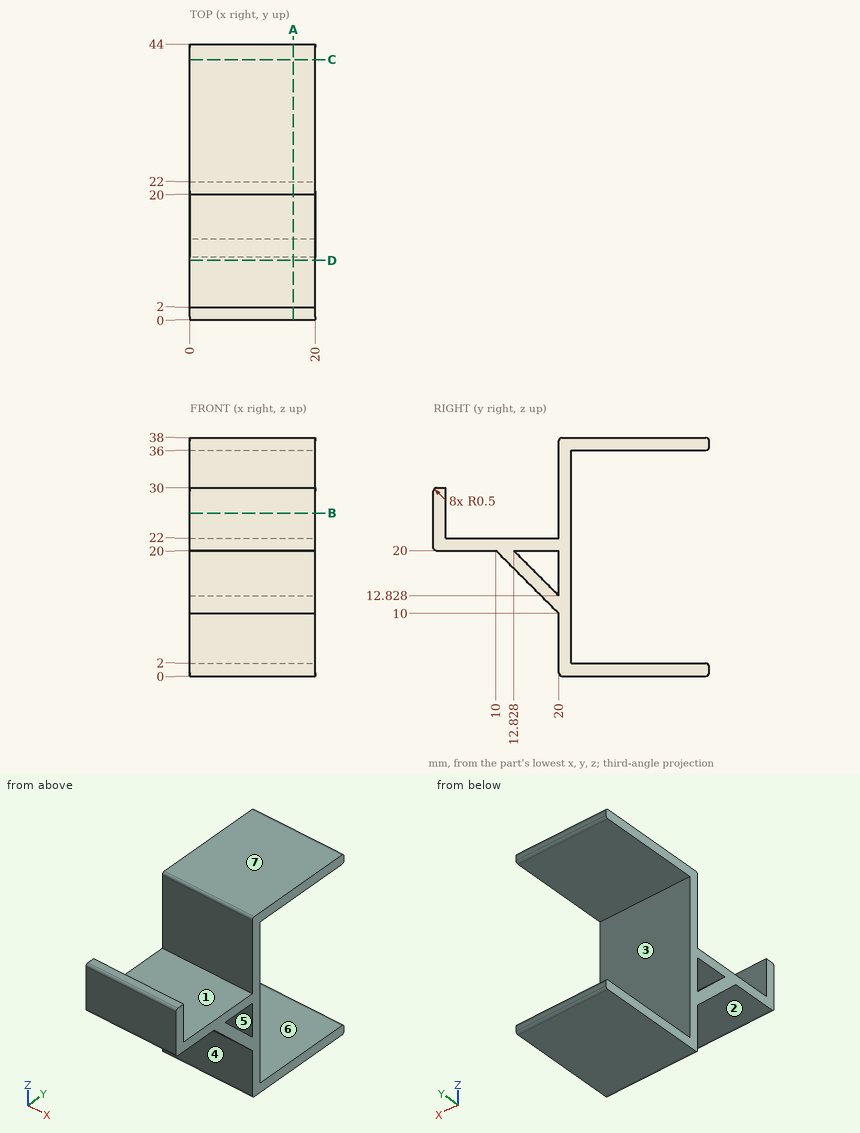
Here's the drawing with two shaded views (mm, measured from the low corner). I have some questions. A direction names the side the tool comes from. Round coordinates to 2 decimals unless told otherwise and drop trailing zeros. Write each loop counter-clockwise with the first axis right and the second up, starting at its lowest first coordinate (ties: lowest second). Pieces come first, ordered by that corner, then holes. Notation, with made-up numbers: M -23,-5 L 32,-5 A22 cw 32,7 Z; hole C -20,-38 d7. An arc over 180 degrees is marked long. Write each question's results on one line, items separated by ' | '. Start each with the question number.
1. Imagine slicing it at D-D on y = 9.5. List the corners of the cut face in (x, z) for me, and give its area (3 significant figures).
2. I need wall thicknesses on L1, parallel to Z at x = 5.25, y = 37.5; L2, parallel to Y at x = 11, z = 29.5; L3, parallel to Y at x = 6.5, z = 4. Which ranges of each line are inside material? Lowest first, please. Write a range as from..to.
3. Imagine slicing it at C-C on y = 41.5. List the corners of the cut face in (x, z) for me.
4. Imagine slicing it at A-A on x = 16.5. List the corners of the cut face in (y, z) for me, and give its area (3 significant figures).
5. Thinking about a two-plate mould opening in Z: for the marked faces 4, 5, 6 and 7, which applies, +Z half, -Z half, draft (parallel to the pull), parting line (faces both ways), or undercut?
6. I'm going to push flat-ended pins straight in: pin 1 Ø12 at (x, z) = (12, 7) entering from -Y; pin 2 Ø4 at (x, z) = (11, 27) entering from +Y; pin 3 Ø5 at (x, y) = (6, 3) entering from -Z. Where does each tip first touch, or does it pass through?
7. Imagine slicing it at B-B on z = 26. List the corners of the cut face in (x, y) for me.
8. On a 3-axis mill with a long thin cutter (end or side, diameter ignored), from which of +Z, -Z, +X, -X, +Y, -Y can I reach the whole of each face in a straight line? I mean the marked faces 1, 2 and 3. Say none if no direction works.
Result sheet:
1) outline: M 0,20 L 20,20 L 20,22 L 0,22 Z | area: 40.0 mm^2
2) L1: z = 0..2, 36..38 | L2: y = 0..2, 20..22 | L3: y = 20..22
3) outline: M 0,0 L 20,0 L 20,2 L 0,2 Z; M 0,36 L 20,36 L 20,38 L 0,38 Z
4) outline: M 0,20.5 A0.5 ccw 0.5,20 L 10,20 L 20,10 L 20,0.5 A0.5 ccw 20.5,0 L 43.5,0 A0.5 ccw 44,0.5 L 44,1.5 A0.5 ccw 43.5,2 L 22,2 L 22,36 L 43.5,36 A0.5 ccw 44,36.5 L 44,37.5 A0.5 ccw 43.5,38 L 20.5,38 A0.5 ccw 20,37.5 L 20,22 L 2,22 L 2,30 L 0.5,30 A0.5 ccw 0,29.5 Z; hole M 12.83,20 L 20,12.83 L 20,20 Z | area: 244 mm^2
5) face 4: draft | face 5: undercut | face 6: undercut | face 7: +Z half
6) pin 1: stops at y = 17 | pin 2: stops at y = 22 | pin 3: stops at z = 20
7) outline: M 0,0 L 20,0 L 20,2 L 0,2 Z; M 0,20 L 20,20 L 20,22 L 0,22 Z
8) face 1: +Z, +X, -X | face 2: -Z, +X, -X, -Y | face 3: +X, -X, +Y
